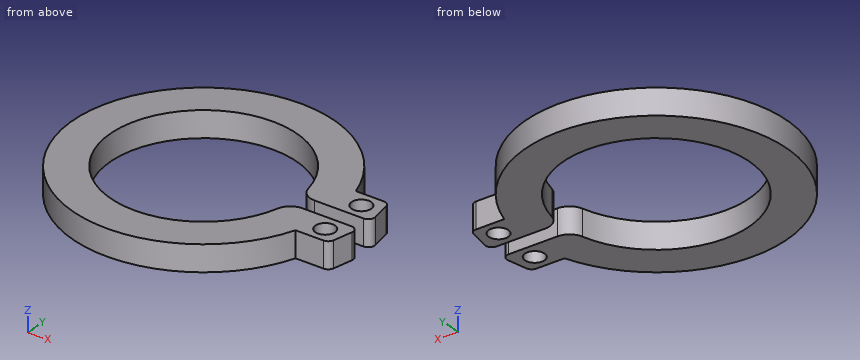
```python
from build123d import *

# Parameters (mm, degrees)
SKETCH1_R           = 0.3
BOSS_EXTRUDE1_DEPTH = 0.4


with BuildPart() as part:
    # Sketch1 → Boss-Extrude1 (new, symmetric)
    with BuildSketch(Plane(origin=(0, 0, 0), x_dir=(0, 1, 0), z_dir=(0, 0, 1))):
        with BuildLine():
            Line((-0.25, -3.264965543), (-0.25, -4.787380599))
            ThreePointArc((-0.25, -4.787380599), (-0.322784356, -4.941705516), (-0.488161799, -4.983706036))
            Line((-0.488161799, -4.983706036), (-1.088161799, -4.86707785))
            ThreePointArc((-1.088161799, -4.86707785), (-1.204324917, -4.797968058), (-1.25, -4.670752414))
            Line((-1.25, -4.670752414), (-1.25, -3.799671038))
            ThreePointArc((-1.25, -3.799671038), (0, 4), (1.25, -3.799671038))
            Line((1.25, -3.799671038), (1.25, -4.670752414))
            ThreePointArc((1.25, -4.670752414), (1.204324917, -4.797968058), (1.088161799, -4.86707785))
            Line((1.088161799, -4.86707785), (0.488161799, -4.983706036))
            ThreePointArc((0.488161799, -4.983706036), (0.322784356, -4.941705516), (0.25, -4.787380599))
            Line((0.25, -4.787380599), (0.25, -3.264965543))
            ThreePointArc((0.25, -3.264965543), (0.358866935, -2.953493353), (0.638059701, -2.777657253))
            ThreePointArc((0.638059701, -2.777657253), (0, 2.85), (-0.638059701, -2.777657253))
            ThreePointArc((-0.638059701, -2.777657253), (-0.358866935, -2.953493353), (-0.25, -3.264965543))
        make_face()
        with Locations(Location((0.75, -4.35, 0), (0, 0, 270))):
            Circle(SKETCH1_R, mode=Mode.SUBTRACT)
        with Locations(Location((-0.75, -4.35, 0), (0, 0, 270))):
            Circle(SKETCH1_R, mode=Mode.SUBTRACT)
    extrude(amount=BOSS_EXTRUDE1_DEPTH, both=True)


solid = part.part
```
Read the model definition and answer for the solid it produces. Units are mm, in the model's axes. Coordinates: 2 decimals unless noted, no trailing zeros. Write each loop counter-clockwise with the first axis right and the second up, starting at its lowest first coordinate (ties: lowest second). Pieces come first, ordered by that corner, then holes. Notation, with made-up numbers: (-28.5, 10) - (-22.5, 10) arc R19 ccw to (-22.5, 28) - close; hole circle Ø3 at (-27.5, 67). An arc over 180 degrees is marked (long way). Answer as a JSON object with one key per item and string values. Group by question number.
1. A cutting plane is placed at A-A (x = 4.35). Determine the outline of the cut face in (y, z), plus the area to 3 significant figures.
2. A cutting plane is placed at D-D (y = -2.25). Determine the outline of the cut face in (x, z), plus the area to 3 significant figures.
3. A cutting plane is placed at C-C (z = -0.2). Determine the outline of the cut face in (x, y), plus the area to 3 significant figures.
4. This flat-tipped pin is pushed along its axis until it touches: P1, Ø2, axis at x = -0.5, y = 0.5, coming from the -Z side. Where does it stop, or does it pass through?
5. A cutting plane is placed at B-B (x = 0). Determine the outline of the cut face in (y, z).
6. Consider L1, parallel to Y at x = 4.35, z = -0.15; L2, parallel to Y at x = 4, z = -0.15; L3, parallel to Y at x = 0.25, z = 0. Determine where each line is inside the solid, lowest interval first. Write a range as [from, to].
Worked out:
{
 "1": {"outline": "(-1.25, -0.4) - (-1.05, -0.4) - (-1.05, 0.4) - (-1.25, 0.4) - close; (-0.45, -0.4) - (-0.25, -0.4) - (-0.25, 0.4) - (-0.45, 0.4) - close; (0.25, -0.4) - (0.45, -0.4) - (0.45, 0.4) - (0.25, 0.4) - close; (1.05, -0.4) - (1.25, -0.4) - (1.25, 0.4) - (1.05, 0.4) - close", "area": "0.640 mm²"},
 "2": {"outline": "(-3.31, -0.4) - (-1.75, -0.4) - (-1.75, 0.4) - (-3.31, 0.4) - close; (1.75, -0.4) - (3.31, -0.4) - (3.31, 0.4) - (1.75, 0.4) - close", "area": "2.49 mm²"},
 "3": {"outline": "(2.78, -0.64) arc R2.85 cw (long way) to (2.78, 0.64) arc R0.5 ccw to (3.26, 0.25) - (4.79, 0.25) arc R0.2 ccw to (4.98, 0.49) - (4.87, 1.09) arc R0.2 ccw to (4.67, 1.25) - (3.8, 1.25) arc R4 ccw (long way) to (3.8, -1.25) - (4.67, -1.25) arc R0.2 ccw to (4.87, -1.09) - (4.98, -0.49) arc R0.2 ccw to (4.79, -0.25) - (3.26, -0.25) arc R0.5 ccw to start; hole circle Ø0.6 at (4.35, -0.75); hole circle Ø0.6 at (4.35, 0.75)", "area": "25.5 mm²"},
 "4": {"P1": "passes through"},
 "5": {"outline": "(-4, -0.4) - (-2.85, -0.4) - (-2.85, 0.4) - (-4, 0.4) - close; (2.85, -0.4) - (4, -0.4) - (4, 0.4) - (2.85, 0.4) - close"},
 "6": {"L1": "y = [-1.25, -1.05], [-0.45, -0.25], [0.25, 0.45], [1.05, 1.25]", "L2": "y = [-1.25, -0.25], [0.25, 1.25]", "L3": "y = [-3.99, -2.84], [2.84, 3.99]"}
}
